Could you check a few things on this model? Use its own coordinates, in mm. Round coordinates to 2 decimals unless told otherwise and drop trailing zeros. Order: outer loops, then holes, each group sorted by start corner. A loop starts at its lowest first (then second) coordinate and runs counter-clockwise, first axis right, second up. Notation, with made-up numbers: M 24.25,63.25 L 29.25,63.25 A33 ccw 29.25,102.25 Z; hole C 15,36 d4. An arc over 180 degrees is marked long. Write each question's results on one line, items separated by ' | '. Start each with the question number.
1. Suppose I cut it at D-D on x = -1. Give the number of separate pieces and of enclosed holes in the cut face, and give its area (3 significant figures).
2. I'm going to push flat-ended pins straight in: pin 1 (4 mm diameter, centred on x = 0, z = 0, fed in from -Y); pin 2 (2 mm diameter, centred on y = 14, z = 6.5, fed in from -X); pin 3 (8 mm diameter, centred on x = -4.5, y = 28.5, fed in from +Z). Where does each tip first touch, or does it pass through?
3. Suppose I cut it at C-C on y = -36.5. Write out the boundary of the cut face in (x, z), and give its area (3 significant figures).
4. Please list where these lines run through material, in increasing order: L1, parallel to Y at x = 3, z = 0; L2, parallel to Z at x = 0, y = -53.75; L3, parallel to Y at x = 3.25, z = 1.
5. Suppose I cut it at A-A on y = 51. Write out the boundary of the cut face in (x, z), and give its area (3 significant figures).
6. Suppose I cut it at B-B on x = 6.5. Write out the boundary of the cut face in (y, z).
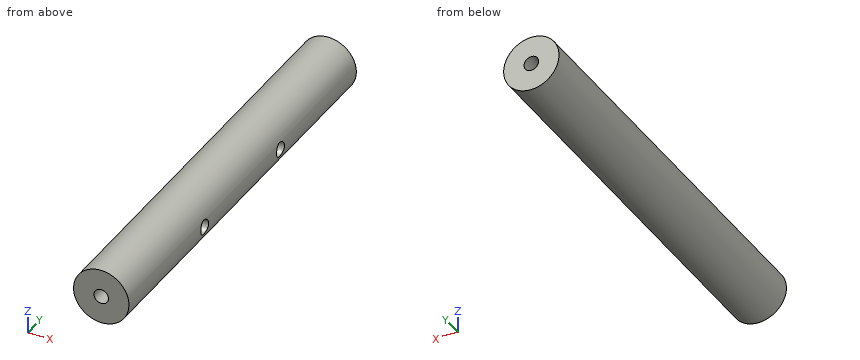
from build123d import *

# Parameters (mm, degrees)
F0_R     = 8
F1_DEPTH = 60
F3_D     = 4.2
F3_DEPTH = 14.4
F3_TIP   = 1.2618073
F5_D     = 4.2
F5_DEPTH = 14.4
F5_TIP   = 1.2618073
F8_D     = 4.2
F8_DEPTH = 14.4
F8_TIP   = 1.2618073


with BuildPart() as f1:
    # F0 (on Front) → F1 (new body, symmetric)
    with BuildSketch(Plane.XZ):
        Circle(F0_R)
    extrude(amount=F1_DEPTH, both=True)

    # F3
    with Locations(Plane.XZ.offset(60)):
        with Locations((0, 0)):
            Hole(F3_D / 2, depth=F3_DEPTH)
            with Locations((0, 0, -(F3_DEPTH + F3_TIP / 2))):  # 118° drill point
                Cone(0, F3_D / 2, F3_TIP, mode=Mode.SUBTRACT)

    # F5
    with Locations(Plane(origin=(0, 60, 0), x_dir=(-1, 0, 0), z_dir=(0, 1, 0))):
        with Locations((0, 0)):
            Hole(F5_D / 2, depth=F5_DEPTH)
            with Locations((0, 0, -(F5_DEPTH + F5_TIP / 2))):  # 118° drill point
                Cone(0, F5_D / 2, F5_TIP, mode=Mode.SUBTRACT)

    # F8
    with Locations(Plane.YZ.offset(8)):
        with Locations((20, 0), (-20, 0)):
            Hole(F8_D / 2, depth=F8_DEPTH)
            with Locations((0, 0, -(F8_DEPTH + F8_TIP / 2))):  # 118° drill point
                Cone(0, F8_D / 2, F8_TIP, mode=Mode.SUBTRACT)


solid = f1.part
Filled sheet:
1) separate pieces: 1 | enclosed holes: 2 | area: 1,770 mm^2
2) pin 1: stops at y = -45.54 | pin 2: stops at x = -5.81 | pin 3: stops at z = 7.98
3) outline: C 0,0 d16 | area: 201 mm^2
4) L1: y = -60 to -22.1, -17.9 to 17.9, 22.1 to 60 | L2: z = -8 to -2.1, 2.1 to 8 | L3: y = -60 to -21.85, -18.15 to 18.15, 21.85 to 60
5) outline: C 0,0 d16; hole C 0,0 d4.2 | area: 187 mm^2
6) outline: M -60,-4.66 L 60,-4.66 L 60,4.66 L -60,4.66 Z; hole C -20,0 d4.2; hole C 20,0 d4.2
